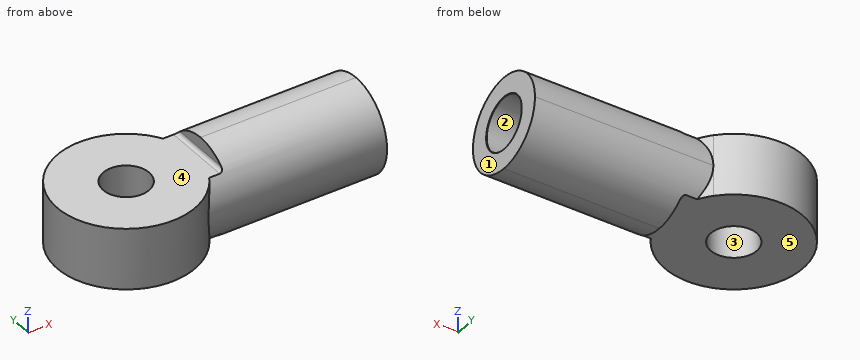
from build123d import *

# Parameters (mm, degrees)
BOSS_EXTRU_2_DEPTH         = 6
ENL_V_START                = -1
ENL_V_MAT_EXTRU_1_DEPTH    = 1
ENL_V_MAT_EXTRU_2_DEPTH    = 1
CONG_4_R                   = 3
CONG_5_R                   = 0.25
D_GAGEMENT_M31_D           = 3.4
D_GAGEMENT_M31_DEPTH       = 5
D_GAGEMENT_M31_CSINK_D     = 3.45
D_GAGEMENT_M31_CSINK_ANGLE = 90
D_GAGEMENT_M31_TIP         = 1.021463052
ESQUISSE9_R                = 1.5
ENL_V_MAT_EXTRU_3_DEPTH    = 17.439282372


with BuildPart() as part:
    # Esquisse1 → Boss.-Extru.2 (new body)
    with BuildSketch(Plane.XY):
        with BuildLine():
            Line((3.354101966, 3), (15, 3))
            Line((15, 3), (15, -3))
            Line((15, -3), (3.354101966, -3))
            ThreePointArc((3.354101966, -3), (-4.5, 0), (3.354101966, 3))
        make_face()
    extrude(amount=BOSS_EXTRU_2_DEPTH)

    # Esquisse5 → Enlèv. mat.-Extru.1 (cut)
    with BuildSketch(Plane.XY.offset(6).offset(ENL_V_START)):
        with BuildLine():
            Line((3.354101966, 3), (4.854101966, 3))
            Line((4.854101966, 3), (4.854101966, -3))
            Line((4.854101966, -3), (3.354101966, -3))
            ThreePointArc((3.354101966, -3), (-4.5, 0), (3.354101966, 3))
        make_face()
    extrude(amount=ENL_V_MAT_EXTRU_1_DEPTH, mode=Mode.SUBTRACT)

    # Esquisse6 → Enlèv. mat.-Extru.2 (cut)
    with BuildSketch(Plane(origin=(0, 0, 0), x_dir=(-1, 0, 0), z_dir=(0, 0, -1))):
        with BuildLine():
            Line((-3.354101966, 3), (-4.854101966, 3))
            Line((-4.854101966, 3), (-4.854101966, -3))
            Line((-4.854101966, -3), (-3.354101966, -3))
            ThreePointArc((-3.354101966, -3), (4.5, 0), (-3.354101966, 3))
        make_face()
    extrude(amount=-ENL_V_MAT_EXTRU_2_DEPTH, mode=Mode.SUBTRACT)

    # Congé4
    # the kernel refuses this fillet: 3 mm, written as the material it takes off along each edge
    with BuildSketch(Plane(origin=(22.5, -3, 6), x_dir=(0, 1, 0), z_dir=(-1, 0, 0))) as cong_4_piece_1_section:
        with BuildLine():
            CenterArc((CONG_4_R, CONG_4_R), CONG_4_R, 180, 90)
            Line((0, CONG_4_R), (0, 0))
            Line((0, 0), (CONG_4_R, 0))
        make_face()
    cong_4_piece_1 = extrude(amount=25.145898034, mode=Mode.PRIVATE)
    cong_4_piece_1 = cong_4_piece_1 - Plane(origin=(0, 0, 5.599963302), x_dir=(0.7453559924999289, -0.6666666666666679, 0), z_dir=(0, 0, -1)) * Cylinder(4.5, 63, mode=Mode.PRIVATE)
    add(cong_4_piece_1, mode=Mode.SUBTRACT)
    with BuildSketch(Plane(origin=(22.5, -3, 0), x_dir=(0, 1, 0), z_dir=(-1, 0, 0))) as cong_4_piece_2_section:
        with BuildLine():
            CenterArc((CONG_4_R, -CONG_4_R), CONG_4_R, 90, 90)
            Line((0, -CONG_4_R), (0, 0))
            Line((0, 0), (CONG_4_R, 0))
        make_face()
    cong_4_piece_2 = extrude(amount=25.145898034, mode=Mode.PRIVATE)
    cong_4_piece_2 = cong_4_piece_2 - Plane(origin=(0, 0, 0.400036698), x_dir=(0.7453559924999289, -0.6666666666666679, 0), z_dir=(0, 0, -1)) * Cylinder(4.5, 63, mode=Mode.PRIVATE)
    add(cong_4_piece_2, mode=Mode.SUBTRACT)
    with BuildSketch(Plane(origin=(-2.645898034, 3, 0), x_dir=(0, 0, 1), z_dir=(1, 0, 0))) as cong_4_piece_3_section:
        with BuildLine():
            CenterArc((CONG_4_R, CONG_4_R), CONG_4_R, 180, 90)
            Line((0, CONG_4_R), (0, 0))
            Line((0, 0), (CONG_4_R, 0))
        make_face()
    cong_4_piece_3 = extrude(amount=25.145898034, mode=Mode.PRIVATE)
    cong_4_piece_3 = cong_4_piece_3 - Plane(origin=(0, 0, 1.508382446), x_dir=(0.7453559924999289, -0.6666666666666679, 0), z_dir=(0, 0, -1)) * Cylinder(4.5, 63, mode=Mode.PRIVATE)
    add(cong_4_piece_3, mode=Mode.SUBTRACT)
    with BuildSketch(Plane(origin=(-2.645898034, 3, 6), x_dir=(0, 0, -1), z_dir=(1, 0, 0))) as cong_4_piece_4_section:
        with BuildLine():
            CenterArc((CONG_4_R, -CONG_4_R), CONG_4_R, 90, 90)
            Line((0, -CONG_4_R), (0, 0))
            Line((0, 0), (CONG_4_R, 0))
        make_face()
    cong_4_piece_4 = extrude(amount=25.145898034, mode=Mode.PRIVATE)
    cong_4_piece_4 = cong_4_piece_4 - Plane(origin=(0, 0, 4.491617554), x_dir=(0.7453559924999289, -0.6666666666666679, 0), z_dir=(0, 0, -1)) * Cylinder(4.5, 63, mode=Mode.PRIVATE)
    add(cong_4_piece_4, mode=Mode.SUBTRACT)

    # Congé5
    cong_5_edges = [part.edges().sort_by_distance(p)[0] for p in [
        (4.854101966, 0, 5),
        (4.854101966, 0, 1),
    ]]
    fillet(cong_5_edges, radius=CONG_5_R)

    # Dégagement M31
    with Locations(Plane(origin=(15, 0, 0), x_dir=(0, 0, -1), z_dir=(1, 0, 0))):
        with Locations((-3, 0)):
            CounterSinkHole(D_GAGEMENT_M31_D / 2, D_GAGEMENT_M31_CSINK_D / 2, depth=D_GAGEMENT_M31_DEPTH, counter_sink_angle=D_GAGEMENT_M31_CSINK_ANGLE)
            with Locations((0, 0, -(D_GAGEMENT_M31_DEPTH + D_GAGEMENT_M31_TIP / 2))):  # 118° drill point
                Cone(0, D_GAGEMENT_M31_D / 2, D_GAGEMENT_M31_TIP, mode=Mode.SUBTRACT)

    # Esquisse9 → Enlèv. mat.-Extru.3 (cut, through all)
    with BuildSketch(Plane.XY.offset(5)):
        Circle(ESQUISSE9_R)
    extrude(amount=-ENL_V_MAT_EXTRU_3_DEPTH, mode=Mode.SUBTRACT)


solid = part.part
Input: part model. Units: mm. Frame: model coordinates. Face numbers are marked on the shaded views. A direction names the side the tool comes from. Coordinates: 2 decimals unless noted, no trailing zeros. Loops run counter-clockwise (first coordinate to the right, second up) from the corner with the lowest first, then second, coordinate; pieces in that order, holes last. Notation, with made-up numbers: (54, -9) -> (75, -9) arc R32 cw to (75, 22) -> close; hole circle Ø8 at (-1, 21.25). An arc over 180 degrees is marked (long way). Write each question's results on one line, items separated by ' | '. Start each with the question number.
Q1. Ray query, line 1 (Z direction, x = 11, y = 0); line 2 (Y direction, x = 12.6, z = 3); line 3 (Z direction, x = 1.75, y = -2). Return the intervals inside material, ascending. Write a range as from..to.
Q2. Pull-direction query (X, two-part tool) for the marked faces 1, 2 and 3; classes: released by +X, released by -X, zero draft, split by the parting line, or undercut.
Q3. Section B-B, the plane x = 13. Return the cut outline in (y, z), plus the area to 3 significant figures.
Q4. Pin query (flat end, axial travel): pin 1 (2.5 mm diameter, centred on x = 0.5, y = -1, fed in from +Z); pin 2 (2.5 mm diameter, centred on x = 0, y = 0.5, fed in from -Z); pin 3 (1 mm diameter, centred on x = 11, z = 4.5, fed in from -Y); pin 4 (2.5 mm diameter, centred on x = 0, y = 0, fed in from +Z). Return the tip coordinate at first contact, or that it passes through.
Q5. Reachability of the marked faces 4 and 5 from +Z, -Z, +X, -X, +Y, -Y: full face, straight path, thin tool, end or side. Return the list, or none.
Q6. Section C-C, the plane x = 6.5. Return the cut outline in (y, z), plus the area to 3 significant figures.
Q7. Section A-A, the plane x = 0. Return the cut outline in (y, z).
Q8. Section D-D, the plane x = -3. Return the cut outline in (y, z), plus the area to 3 significant figures.
Found:
1) line 1: 0..1.3, 4.7..6 | line 2: -3..-1.7, 1.7..3 | line 3: 1..5
2) face 1: released by +X | face 2: zero draft | face 3: undercut
3) outline: circle Ø6 at (0, 3); hole circle Ø3.4 at (0, 3) | area: 19.2 mm2
4) pin 1: z = 5 | pin 2: z = 1 | pin 3: y = -2.83 | pin 4: through
5) face 4: +Z, -X, +Y, -Y | face 5: -Z, -X, +Y, -Y
6) outline: circle Ø6 at (0, 3) | area: 28.3 mm2
7) outline: (-4.5, 1) -> (-1.5, 1) -> (-1.5, 5) -> (-4.5, 5) -> close; (1.5, 1) -> (4.5, 1) -> (4.5, 5) -> (1.5, 5) -> close
8) outline: (-3.35, 1) -> (3.35, 1) -> (3.35, 5) -> (-3.35, 5) -> close | area: 26.8 mm2
